Autodesk Inventor part; units mm, degrees
ref_plane "YZ Plane" through (0, 0, 0) normal (1, 0, 0) x (0, 1, 0)
ref_plane "XZ Plane" through (0, 0, 0) normal (0, 1, 0) x (-1, 0, 0)
ref_plane "XY Plane" through (0, 0, 0) normal (0, 0, 1) x (1, 0, 0)
sketch "Sketch1" plane through (0, 0, 0) normal (0, 0, 1) x (1, 0, 0)
  line L0 (-7.9197, 10.2868) -> (-22.9197, 10.2868)
  line L1 (-22.9197, 10.2868) -> (-22.9197, -14.7132)
  line L2 (-22.9197, -14.7132) -> (-7.9197, -14.7132)
  line L3 (-7.9197, -14.7132) -> (-7.9197, 10.2868)
  point P0 (0, 0)
  dimension "d0" = 15
  dimension "d1" = 25
extrude "Extrusion1" add sketch "Sketch1" along normal blind 1
sketch "Sketch2" plane through (0, 0, 1) normal (0, 0, 1) x (1, 0, 0)
  circle A0 centre (-17.8268, 6.422) radius 2.5
  circle A1 centre (-17.8268, -7.5909) radius 2.5
  point P0 (0, 0)
  dimension "d4" = 5
  dimension "d5" = 5
hole "Hole1" at (-17.8268, 6.422, 1) at (-17.8268, -7.5909, 1) direction (0, 0, -1) diameter 3 end through all
sketch "Sketch3" plane through (0, 0, 1) normal (0, 0, 1) x (1, 0, 0)
  line L0 (-22.9197, -14.7132) -> (-7.9197, -14.7132)
  line L1 (-7.9197, 10.2868) -> (-22.9197, 10.2868)
  line L2 (-7.9197, -14.7132) -> (-7.9197, 10.2868)
  line L3 (-8.5412, 9.8751) -> (-7.9197, 9.8751)
  line L4 (-7.9197, 9.8751) -> (-7.9197, -14.2385)
  line L5 (-7.9197, -14.2385) -> (-8.5412, -14.2385)
  line L6 (-8.5412, -14.2385) -> (-8.5412, 9.8751)
  point P0 (0, 0)
  dimension "d13" = 25
  dimension "d14" = 15
extrude "Extrusion2" add sketch "Sketch3" along normal blind 15
sketch "Sketch4" plane through (-8.5412, -14.2385, 1) normal (-1, 0, 0) x (0, 0, 1)
  circle A0 centre (5.1833, 19.9887) radius 2.5
  circle A1 centre (7.6833, 6.1285) radius 2.5
  point P0 (-1, 14.2385)
  dimension "d17" = 5
  dimension "d18" = 5
hole "Hole2" at (-8.5412, 5.7501, 6.1833) at (-8.5412, -8.1101, 8.6833) direction (1, 0, 0) diameter 3 end through all
properties part number "L angle"
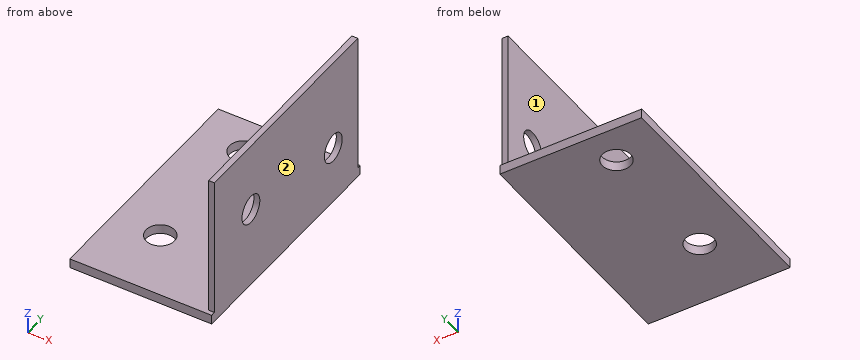
Source: CAD feature listing. Evaluate the final solid. Frame: model axes, mm. Face numbers are marked on the shaded views. A direction names the side the tool comes from. Coordinates: 2 decimals unless noted, no trailing zeros. Write each loop counter-clockwise with the first axis right and the second up, starting at its lowest first coordinate (ties: lowest second). Pieces come first, ordered by that corner, then holes. Notation, with made-up numbers: M 24,64.5 L 65,64.5 A11 ccw 65,81.5 Z; hole C 15,13 d1. An arc over 180 degrees is marked long. Use a Markdown table: item, result.
1) Section D-D, the plane x = -9.5. Output: boundary loops of the cut face in (y, z).
Conclusion:
| item | result |
|---|---|
| outline | M -14.71,0 L 10.29,0 L 10.29,1 L -14.71,1 Z |
2) Section B-B, the plane y = -3. Output: boundary loops of the cut face in (x, z).
Conclusion:
| item | result |
|---|---|
| outline | M -22.92,0 L -7.92,0 L -7.92,16 L -8.54,16 L -8.54,1 L -22.92,1 Z |
3) Section A-A, the plane z = 8.5. Output: boundary loops of the cut face in (x, y).
Conclusion:
| item | result |
|---|---|
| outline | M -8.54,-14.24 L -7.92,-14.24 L -7.92,-9.6 L -8.54,-9.6 Z; M -8.54,-6.62 L -7.92,-6.62 L -7.92,9.88 L -8.54,9.88 Z |
4) Reachability of the marked faces 1 and 2 from +Z, -Z, +X, -X, +Y, -Y: full face, straight path, thin tool, end or side. Return the list, or none.
Conclusion:
| item | result |
|---|---|
| face 1 | +Z, -X, +Y, -Y |
| face 2 | +Z, -Z, +X, +Y, -Y |
5) Ray query, L1, parallel to Z at x = -14.25, y = -4.75; L2, parallel to X at y = -8.75, z = 14. Return the intervals inside material, ascending.
Conclusion:
| item | result |
|---|---|
| L1 | z = 0 to 1 |
| L2 | x = -8.54 to -7.92 |
6) Section C-C, the plane z = 14. Output: boundary loops of the cut face in (x, y), then the cut area to 3 significant figures.
Conclusion:
| item | result |
|---|---|
| outline | M -8.54,-14.24 L -7.92,-14.24 L -7.92,9.88 L -8.54,9.88 Z |
| area | 15.0 mm^2 |
7) First-contact query: pin 1 Ø1.5 at (x, y) = (-21, 4.5) entering from +Z; pin 2 Ø3 at (x, z) = (-10, 6) entering from +Y; pin 3 Ø4 at (y, z) = (-8.11, 8.68) entering from -X. Flat tips, straight axial feed; report the tip coordinate or a pass-through.
Conclusion:
| item | result |
|---|---|
| pin 1 | stops at z = 1 |
| pin 2 | stops at y = 9.88 |
| pin 3 | stops at x = -8.54 |
